Part print with two shaded views. Sizes in mm from the minimum x, y, z corner. A direction names the side the tool comes from. Give positions to 0.01 mm unless a question says otherwise; leave off trailing zeros. Write each loop counter-clockwise with the first axis right and the second up, starting at its lowest first coordinate (ties: lowest second). Pieces come first, ordered by that corner, then holes. Notation, with made-up numbers: (5.25, 70.25) - (34.25, 70.25) arc R33 ccw to (34.25, 105.25) - close; hole circle Ø8 at (44.5, 72.25). An arc over 180 degrees is marked (long way). Answer as a JSON object with one key per item and string values.
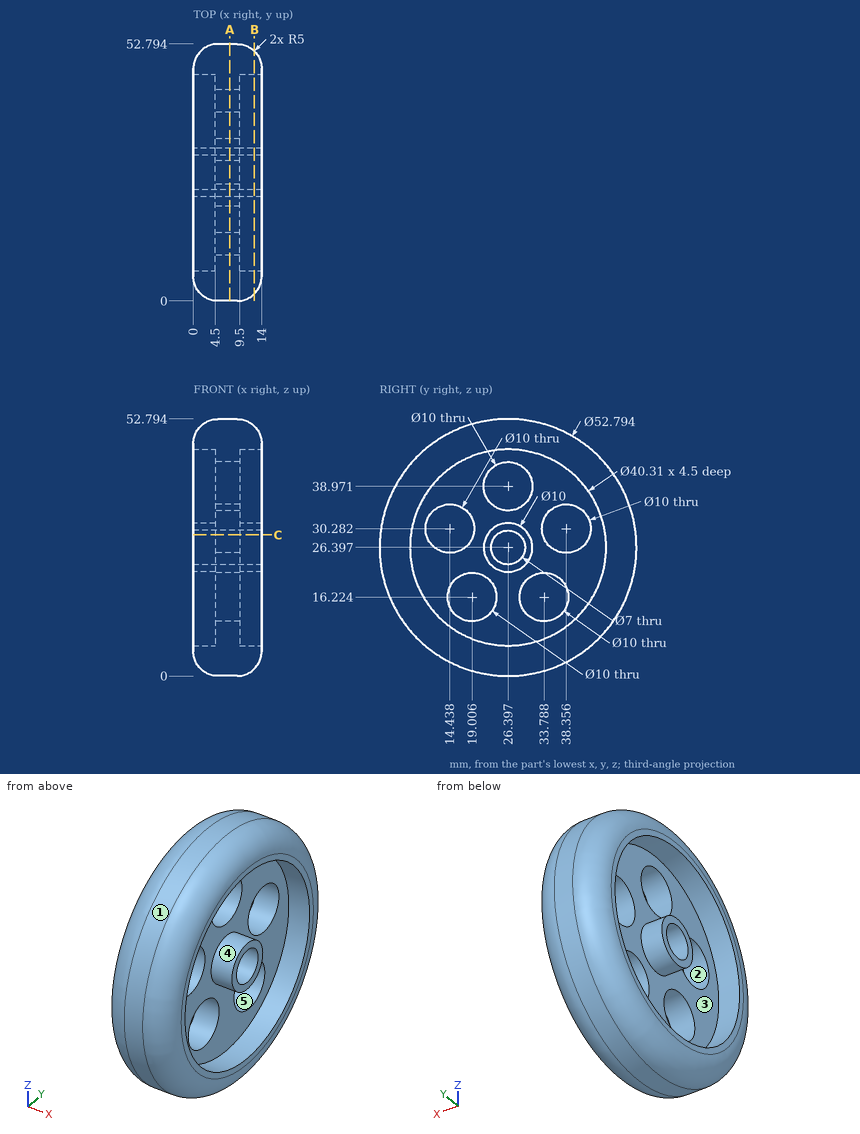
(1) Saw through at C-C, the plane z = 29. State how many separate pieces and enclosed holes the cut face has, and give its area (3 significant figures).
Answer key:
{"separate pieces": "4", "enclosed holes": "0", "area": "269 mm²"}
(2) Pull direction Y, two halves, no side cores. Call the marked faces 1 and 2: pulls with the +Y half, pulls with the -Y half, needs draft (parallel to the pull), parting line crosses it, or undercut.
Answer key:
{"face 1": "parting line crosses it", "face 2": "undercut"}
(3) Flat gauge pins, fed straight in: P1, Ø11.5, axis at y = 38.36, z = 30.28, coming from the +X side; P2, Ø3, axis at x = 7.5, y = 27, coming from the -Z side; P3, Ø1, axis at x = 12.5, z = 32.5, coming from the +Y side; P4, Ø3, axis at x = 6.5, z = 15.5, coming from the -Y side. Where does each tip first touch, or does it go through?
Answer key:
{"P1": "stops at x = 9.5", "P2": "stops at z = 0", "P3": "stops at y = 51.07", "P4": "stops at y = 1.73"}
(4) Saw through at B-B, the plane x = 12.5. Give the cut face in (y, z) (1 decimal).
Answer key:
{"outline": "circle Ø49.9 at (26.4, 26.4); circle Ø10 at (26.4, 26.4); hole circle Ø40.3 at (26.4, 26.4); hole circle Ø7 at (26.4, 26.4)"}
(5) 3-axis set-ups, long thin cutter, end or side, ignore diameter. For the marked faces 3, 4 and 5: which of +Z, -Z, +X, -X, +Y, -Y reach the whole face in a straight line?
Answer key:
{"face 3": "-X", "face 4": "+X", "face 5": "+X, -X"}
(6) Probe L1, parallel to Z at x = 4.75, y = 37 (1 decimal); L2, parallel to Z at x = 5.5, y = 36 (1 decimal); L3, parallel to Y at x = 10.5, z = 29 (1 decimal). List the from-to ranges inside material, lowest first. Write a range as [from, to].
Answer key:
{"L1": "z = [2.2, 12.4], [20.1, 25.5], [35.1, 50.6]", "L2": "z = [1.8, 11.7], [20.7, 25.9], [34.7, 51]", "L3": "y = [0.4, 6.4], [22.1, 24.1], [28.7, 30.7], [46.4, 52.4]"}
(7) Saw through at A-A, the plane x = 7.5. Give the cut face in (y, z) (1 decimal).
Answer key:
{"outline": "circle Ø52.8 at (26.4, 26.4); hole circle Ø10 at (14.4, 30.3); hole circle Ø10 at (19, 16.2); hole circle Ø10 at (26.4, 39); hole circle Ø7 at (26.4, 26.4); hole circle Ø10 at (33.8, 16.2); hole circle Ø10 at (38.4, 30.3)"}
